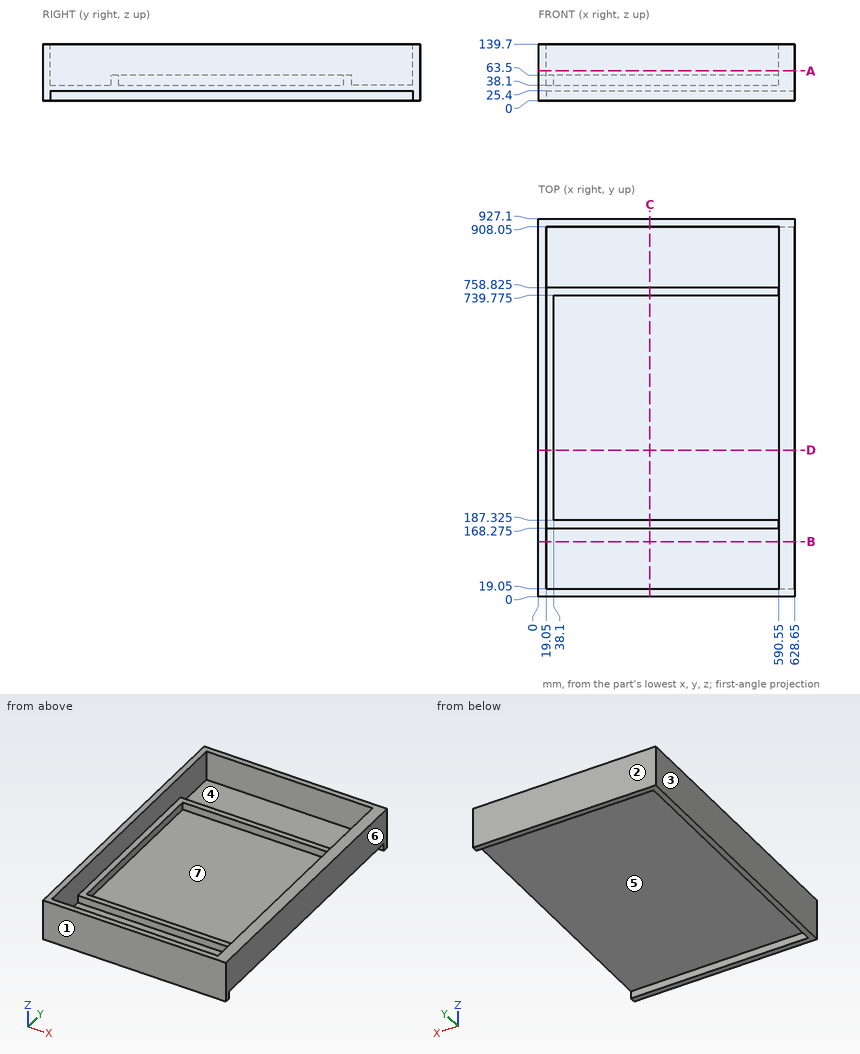
Check sheet for the drawn part. Datum: minimum x, y, z corner. Units: mm. A direction names the side the tool comes from. Round coordinates to 2 decimals unless told otherwise and drop trailing zeros. Order: outer loops, then holes, each group sorted by start corner. A loop starts at its lowest first (then second) coordinate and runs counter-clockwise, first axis right, second up.
1) Section check A-A (z = 74). Record the boundary of the cut face in (x, y), and give its area (3 significant figures).
2) Tool access check on the marked faces 5, 6 and 7. Record the directions out of +Z, -Z, +X, -X, +Y, -Y that give a thin tool (end or side, any length) a straight path to the whole face; none if there is none.
3) Go/stop test with flat-tipped pins: pin 1 Ø12 at (x, y) = (137.5, 357.5) entering from -Z; pin 2 Ø7.5 at (y, z) = (571, 17) entering from +X; pin 3 Ø2 at (x, y) = (521.5, 469.5) entering from +Z. Record where each tip stops, or that it passes through.
4) Mould release check, pull along Y, two halves, no side actions. Record for the marked faces 1, 2, 3 and 4: +Y half, -Y half, draft (parallel to the pull), parting line (faces both ways), or undercut.
5) Scan lines: line 1 (Y direction, x = 354.5, z = 39.5) (3 decimals); line 2 (X direction, y = 63, z = 49.5); line 3 (X direction, y = 633.5, z = 43). Record each from-to range of solid material in increasing order.
6) Section check B-B (y = 135.5). Record the boundary of the cut face in (x, z).
7) Section check D-D (y = 360). Record the boundary of the cut face in (x, z), and give its area (3 significant figures).
8) Section check C-C (x = 274). Record the boundary of the cut face in (y, z) (3 decimals), and give its area (3 significant figures).
Result:
1. outline: (0, 0) - (628.65, 0) - (628.65, 927.1) - (0, 927.1) - close; hole (19.05, 19.05) - (590.55, 19.05) - (590.55, 908.05) - (19.05, 908.05) - close
1. area: 74,800 mm2
2. face 5: -Z, +X
2. face 6: +Z, -Z, +X, +Y, -Y
2. face 7: +Z
3. pin 1: stops at z = 25.4
3. pin 2: stops at x = 19.05
3. pin 3: stops at z = 38.1
4. face 1: -Y half
4. face 2: +Y half
4. face 3: draft
4. face 4: undercut
5. line 1: y = 0 to 19.05, 168.275 to 187.325, 739.775 to 758.825, 908.05 to 927.1
5. line 2: x = 0 to 19.05, 590.55 to 628.65
5. line 3: x = 0 to 38.1, 590.55 to 628.65
6. outline: (0, 0) - (19.05, 0) - (19.05, 25.4) - (628.65, 25.4) - (628.65, 139.7) - (590.55, 139.7) - (590.55, 38.1) - (19.05, 38.1) - (19.05, 139.7) - (0, 139.7) - close
7. outline: (0, 0) - (19.05, 0) - (19.05, 25.4) - (628.65, 25.4) - (628.65, 139.7) - (590.55, 139.7) - (590.55, 38.1) - (38.1, 38.1) - (38.1, 63.5) - (19.05, 63.5) - (19.05, 139.7) - (0, 139.7) - close
7. area: 14,800 mm2
8. outline: (0, 0) - (19.05, 0) - (19.05, 25.4) - (908.05, 25.4) - (908.05, 0) - (927.1, 0) - (927.1, 139.7) - (908.05, 139.7) - (908.05, 38.1) - (758.825, 38.1) - (758.825, 63.5) - (739.775, 63.5) - (739.775, 38.1) - (187.325, 38.1) - (187.325, 63.5) - (168.275, 63.5) - (168.275, 38.1) - (19.05, 38.1) - (19.05, 139.7) - (0, 139.7) - close
8. area: 17,600 mm2
